```python
from build123d import *

# Parameters (mm, degrees)
SWEEP_1_PROFILE_R         = 1
SKETCH_9_R                = 9
EXTRUDE_1_DEPTH           = 3
EXTRUDE_1_TAPER           = 60
EXTRUDE_1_OTHER_WAY_DEPTH = 3


with BuildPart() as part:
    # 扫描1: sweep along a path in 草图1
    with BuildLine(Plane.XY) as sweep_1_path:
        Line((8, 4), (-8, 4))
        ThreePointArc((-8, 4), (-12, 0), (-8, -4))
        Line((-8, -4), (8, -4))
        ThreePointArc((8, -4), (12, 0), (8, 4))
    # 扫描1 profile (on start of the path) → 扫描1 (sweep)
    with BuildSketch(Plane(origin=(8, 4, 0), x_dir=(0, 0, -1), z_dir=(-1, 0, 0))):
        Circle(SWEEP_1_PROFILE_R)
    sweep(path=sweep_1_path.line)

    # 草图9 → 凸台-拉伸1 (add)
    with BuildSketch(Plane(origin=(0, 0, 0), x_dir=(0, 0, -1), z_dir=(1, 0, 0))):
        Circle(SKETCH_9_R)
    extrude(amount=EXTRUDE_1_DEPTH, taper=EXTRUDE_1_TAPER)

    # 草图9 → 凸台-拉伸1 other way (add)
    with BuildSketch(Plane(origin=(0, 0, 0), x_dir=(0, 0, -1), z_dir=(1, 0, 0))):
        Circle(SKETCH_9_R)
    extrude(amount=-EXTRUDE_1_OTHER_WAY_DEPTH)


solid = part.part
```
Here's how the part is built. I have some questions about the finished solid (model axes, mm). Give positions to 0.01 mm unless a question says otherwise; leave off trailing zeros. Order: outer loops, then holes, each group sorted by start corner. A loop starts at its lowest first (then second) coordinate and runs counter-clockwise, first axis right, second up. Notation, with made-up numbers: M 43.5,36 L 86.5,36 A34 cw 86.5,72 Z; hole C 83.5,50 d8. An arc over 180 degrees is marked long. Use a Markdown table: item, result. Add a question column.
1. For pin 1 Ø4 at (y, z) = (-0.5, 7) entering from +X; pin 2 Ø10 at (x, y) = (10.5, -6) entering from +Z; pin 3 Ø6 at (x, z) = (-8.5, 0) entering from -Y, each with a flat end and sliding along its axis, tell me the tip position at first contact or that it passes through.
2. Suppose I cut it at B-B (x = -4). List the corners of the cut face in (y, z) for me, and give its area (3 significant figures).
3. I need wall thicknesses on probe 1 along Y at (x, z) = (3.25, 0.5); probe 2 along X at (y, z) = (1.5, 6); probe 3 along X at (y, z) = (-2.75, -2.5). Which ranges of each line are inside material? Lowest first, please. Write a range as from..to.
4. Suppose I cut it at C-C (y = 0). Give the number of separate pieces and of enclosed holes in the cut face, and give its area (3 significant figures).
5. Suppose I cut it at A-A (z = 0). List the corners of the cut face in (x, y) for me.
6. Suppose I cut it at D-D (x = 2). List the corners of the cut face in (y, z) for me, and give its area (3 significant figures).
7. If we mould it in two halves opening along X, with no side actions, what happens to faces 1 (the cylindrical face through (-5, -3, 0)), 2 (the cylindrical face through (5, -5, 0)), 3 (the cylindrical face through (-1.479, 8.923, 1.172))? For each: +X half, -X half, draft (parallel to the pull), parting line (faces both ways), or undercut.
Results list:
| question | item | result |
|---|---|---|
| 1 | pin 1 | stops at x = 2.3 |
| 1 | pin 2 | stops at z = 1 |
| 1 | pin 3 | stops at y = -5 |
| 2 | outline | C -4,0 d2; C 4,0 d2 |
| 2 | area | 6.28 mm² |
| 3 | probe 1 | y = -4.87..-3.13, 3.13..4.87 |
| 3 | probe 2 | x = -3..1.63 |
| 3 | probe 3 | x = -3..3 |
| 4 | separate pieces | 3 |
| 4 | enclosed holes | 0 |
| 4 | area | 98.7 mm² |
| 5 | outline | M -8,-5 L -3,-5 L -3,-9 L 0,-9 L 2.31,-5 L 8,-5 A5 ccw 8,5 L 2.31,5 L 0,9 L -3,9 L -3,5 L -8,5 A5 ccw Z; hole M -8,-3 L -3,-3 L -3,3 L -8,3 A3 ccw Z; hole M 3,-3 L 8,-3 A3 ccw 8,3 L 3,3 Z |
| 6 | outline | C 0,0 d11.07 |
| 6 | area | 96.3 mm² |
| 7 | face 1 | undercut |
| 7 | face 2 | undercut |
| 7 | face 3 | draft |
